Geometry check sheet. Reference: the model listing, model coordinates, mm. Face numbers are marked on the shaded views. A direction names the side the tool comes from. Coordinates: 2 decimals unless noted, no trailing zeros. Order: outer loops, then holes, each group sorted by start corner. A loop starts at its lowest first (then second) coordinate and runs counter-clockwise, first axis right, second up. Notation, with made-up numbers: (-16.75, 24) -> (-8.75, 24) arc R29 cw to (-8.75, 56) -> close; hole circle Ø5 at (85, 7.5). An arc over 180 degrees is marked (long way). Answer as CSV lines item,"result". Start each with the question number.
from build123d import *

# Parameters (mm, degrees)
SKETCH1_R           = 0.75
BOSS_EXTRUDE1_DEPTH = 2


with BuildPart() as part:
    # Sketch1 → Boss-Extrude1 (new body)
    with BuildSketch(Plane.XY):
        with BuildLine():
            Line((0, 14.74), (0, 7))
            Line((0, 7), (4, 7))
            Line((4, 7), (4, 5))
            Line((4, 5), (0, 5))
            Line((0, 5), (0, 2))
            ThreePointArc((0, 2), (0.585786438, 0.585786438), (2, 0))
            Line((2, 0), (14.2, 0))
            ThreePointArc((14.2, 0), (15.614213562, 0.585786438), (16.2, 2))
            Line((16.2, 2), (16.2, 5))
            Line((16.2, 5), (12.2, 5))
            Line((12.2, 5), (12.2, 7))
            Line((12.2, 7), (16.2, 7))
            Line((16.2, 7), (16.2, 14.74))
            Line((16.2, 14.74), (12.2, 14.74))
            Line((12.2, 14.74), (12.2, 16.74))
            Line((12.2, 16.74), (16.2, 16.74))
            Line((16.2, 16.74), (16.2, 19.74))
            ThreePointArc((16.2, 19.74), (15.614213562, 21.154213562), (14.2, 21.74))
            Line((14.2, 21.74), (2, 21.74))
            ThreePointArc((2, 21.74), (0.585786438, 21.154213562), (0, 19.74))
            Line((0, 19.74), (0, 16.74))
            Line((0, 16.74), (4, 16.74))
            Line((4, 16.74), (4, 14.74))
            Line((4, 14.74), (0, 14.74))
        make_face()
        with Locations((13.45, 2.5)):
            Circle(SKETCH1_R, mode=Mode.SUBTRACT)
        with Locations((2.75, 19.24)):
            Circle(SKETCH1_R, mode=Mode.SUBTRACT)
        with Locations((2.75, 2.5)):
            Circle(SKETCH1_R, mode=Mode.SUBTRACT)
        with Locations((13.45, 19.24)):
            Circle(SKETCH1_R, mode=Mode.SUBTRACT)
    extrude(amount=BOSS_EXTRUDE1_DEPTH)


solid = part.part
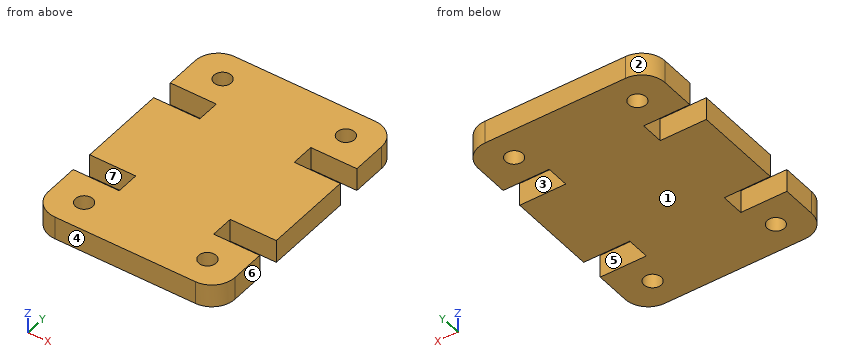
Q1. Sectioned sample at B-B, the plane x = 13.45. Record the cut outline in (y, z).
Q2. Go/stop test with flat-tipped pins: pin 1 Ø0.6 at (y, z) = (16, 1.5) entering from +X; pin 2 Ø1.2 at (x, y) = (2.75, 2.5) entering from +Z. Record where each tip stops, or that it passes through.
Q3. Release check for a two-part mould opening along Y. For the marked faces 1, 2, 3 and 4 record: released by +Y, released by -Y, zero draft, split by the parting line, or undercut.
Q4. Sectioned sample at A-A, the plane y = 19.24. Record the cut outline in (x, z), then the cut area to 3 significant figures.
Q5. Sectioned sample at C-C, the plane x = 1.5. Record the cut outline in (y, z).
Q6. Thickness scan on L1, parallel to Y at x = 12.25, z = 1.2; L2, parallel to Y at x = 13.45, z = 1.1; L3, parallel to X at y = 6.25, z = 1.5. Record the ranges inside material, lowest first.
Q7. Access from +Z, -Z, +X, -X, +Y, -Y to the whole of each face (thin tool, end or side, straight path). Record for the marked faces 5, 6 and 7.
Geometry results:
1,outline,"(0, 0) -> (1.75, 0) -> (1.75, 2) -> (0, 2) -> close; (3.25, 0) -> (5, 0) -> (5, 2) -> (3.25, 2) -> close; (7, 0) -> (14.74, 0) -> (14.74, 2) -> (7, 2) -> close; (16.74, 0) -> (18.49, 0) -> (18.49, 2) -> (16.74, 2) -> close; (19.99, 0) -> (21.74, 0) -> (21.74, 2) -> (19.99, 2) -> close"
2,pin 1,"stops at x = 12.2"
2,pin 2,"passes through"
3,face 1,"zero draft"
3,face 2,"released by +Y"
3,face 3,"undercut"
3,face 4,"released by -Y"
4,outline,"(0, 0) -> (2, 0) -> (2, 2) -> (0, 2) -> close; (3.5, 0) -> (12.7, 0) -> (12.7, 2) -> (3.5, 2) -> close; (14.2, 0) -> (16.2, 0) -> (16.2, 2) -> (14.2, 2) -> close"
4,area,"26.4 mm^2"
5,outline,"(0.06, 0) -> (5, 0) -> (5, 2) -> (0.06, 2) -> close; (7, 0) -> (14.74, 0) -> (14.74, 2) -> (7, 2) -> close; (16.74, 0) -> (21.68, 0) -> (21.68, 2) -> (16.74, 2) -> close"
6,L1,"y = 0 to 5, 7 to 14.74, 16.74 to 21.74"
6,L2,"y = 0 to 1.75, 3.25 to 5, 7 to 14.74, 16.74 to 18.49, 19.99 to 21.74"
6,L3,"x = 4 to 12.2"
7,face 5,"+Z, -Z, +X"
7,face 6,"+Z, -Z, +X, +Y, -Y"
7,face 7,"+Z, -Z, -X"
